```python
from build123d import *

# Parameters (mm, degrees)
F0_W     = 10
F0_H     = 15
F0_R     = 6
F0_R_2   = 3
F1_DEPTH = 20
F2_DEPTH = 75
F3_DEPTH = 10
F4_R     = 3
F5_DEPTH = 113.001
F6_R     = 5


with BuildPart() as f1:
    # F0 (on Top) → F1 (new body)
    with BuildSketch(Plane.XY):
        with Locations((-51.5, 0)):
            Rectangle(F0_W, F0_H)
        with BuildLine():
            ThreePointArc((-15.8113883008, -7.5), (-17.5, 0), (-15.8113883008, 7.5))
            Line((-15.8113883008, 7.5), (-46.5, 7.5))
            Line((-46.5, 7.5), (-46.5, -7.5))
            Line((-46.5, -7.5), (-15.8113883008, -7.5))
        make_face()
        with BuildLine():
            ThreePointArc((15.8113883008, -7.5), (17.0726286093, -3.843872054), (17.5, 0))
            ThreePointArc((17.5, 0), (17.0726286093, 3.843872054), (15.8113883008, 7.5))
            Line((15.8113883008, 7.5), (-15.8113883008, 7.5))
            ThreePointArc((-15.8113883008, 7.5), (-17.5, 0), (-15.8113883008, -7.5))
            Line((-15.8113883008, -7.5), (15.8113883008, -7.5))
        make_face()
        Circle(F0_R, mode=Mode.SUBTRACT)
        with BuildLine():
            Line((-15.8113883008, 7.5), (15.8113883008, 7.5))
            ThreePointArc((15.8113883008, 7.5), (0, 17.5), (-15.8113883008, 7.5))
        make_face()
        with BuildLine():
            ThreePointArc((-15.8113883008, -7.5), (0, -17.5), (15.8113883008, -7.5))
            Line((15.8113883008, -7.5), (-15.8113883008, -7.5))
        make_face()
        Circle(F0_R)
        Circle(F0_R_2, mode=Mode.SUBTRACT)
        with BuildLine():
            ThreePointArc((15.8113883008, 7.5), (17.0726286093, 3.843872054), (17.5, 0))
            ThreePointArc((17.5, 0), (17.0726286093, -3.843872054), (15.8113883008, -7.5))
            Line((15.8113883008, -7.5), (46.5, -7.5))
            Line((46.5, -7.5), (46.5, 7.5))
            Line((46.5, 7.5), (15.8113883008, 7.5))
        make_face()
        with Locations((51.5, 0)):
            Rectangle(F0_W, F0_H)
    extrude(amount=F1_DEPTH)

    # F0 (on Top) → F2 (join)
    with BuildSketch(Plane.XY):
        with Locations((-51.5, 0)):
            Rectangle(F0_W, F0_H)
        with Locations((51.5, 0)):
            Rectangle(F0_W, F0_H)
    extrude(amount=-F2_DEPTH)

    # F0 (on Top) → F3 (cut)
    with BuildSketch(Plane.XY):
        Circle(F0_R)
        Circle(F0_R_2, mode=Mode.SUBTRACT)
    extrude(amount=F3_DEPTH, mode=Mode.SUBTRACT)

    # F4 (on face) → F5 (cut, through all)
    with BuildSketch(Plane.YZ.offset(56.5)):
        with BuildLine():
            Line((7.5, -75), (7.5, -67.5))
            ThreePointArc((7.5, -67.5), (5.3033008589, -72.8033008589), (0, -75))
            Line((0, -75), (7.5, -75))
        make_face()
        with BuildLine():
            Line((-7.5, -75), (0, -75))
            ThreePointArc((0, -75), (-5.3033008589, -72.8033008589), (-7.5, -67.5))
            Line((-7.5, -67.5), (-7.5, -75))
        make_face()
        with Locations((0, -67.5)):
            Circle(F4_R)
    extrude(amount=-F5_DEPTH, mode=Mode.SUBTRACT)

    # F6
    f6_edges = [f1.edges().sort_by_distance(p)[0] for p in [
        (-36.155694, -7.5, 20),
        (-56.5, -7.5, -23.75),
        (56.5, -7.5, -23.75),
        (36.155694, -7.5, 20),
        (56.5, 0, 20),
        (-56.5, 0, 20),
        (-36.155694, 7.5, 20),
        (36.155694, 7.5, 20),
        (0, -17.5, 0),
        (-31.155694, -7.5, 0),
        (31.155694, -7.5, 0),
        (-31.155694, 7.5, 0),
        (31.155694, 7.5, 0),
        (0, 17.5, 0),
    ]]
    fillet(f6_edges, radius=F6_R)


solid = f1.part
```
Here's how the part is built. I have some questions about the finished solid (model axes, mm). A direction names the side the tool comes from. Round coordinates to 2 decimals unless told otherwise and drop trailing zeros. Loops run counter-clockwise (first coordinate to the right, second up) from the corner with the lowest first, then second, coordinate; pieces in that order, holes last.
1. For faces 1 (the face through (29.13, 6, 1.43)), 2 (the face through (47, 7.5, -14)), 3 (the face through (-47, -7.5, -14)), which set-ups out of +Z, -Z, +X, -X, +Y, -Y let a thin tool reach every point of the face, with its end or its side?
Answers:
face 1: -Z, +Y
face 2: +Z, -Z, +X, +Y
face 3: +Z, -Z, -X, -Y
2. Thinking about a two-plate mould opening in Y: for faces 4 (the face through (-29.13, -6, 1.43)), 5 (the face through (-3, -1, 10)), 6 (the face through (0.35, 17.497, 12.395)), which applies, released by +Y, released by -Y, zero draft, split by the parting line, or undercut?
Answers:
face 4: released by -Y
face 5: undercut
face 6: released by +Y
3. Suppose I cut it at B-B, the plane z = -59.5. Please give me the cut outline in (x, y).
Answers:
outline: (-56.5, -2.5) arc R5 ccw to (-51.5, -7.5) - (-46.5, -7.5) - (-46.5, 7.5) - (-51.5, 7.5) arc R5 ccw to (-56.5, 2.5) - close; (46.5, -7.5) - (51.5, -7.5) arc R5 ccw to (56.5, -2.5) - (56.5, 2.5) arc R5 ccw to (51.5, 7.5) - (46.5, 7.5) - close
4. Suppose I cut it at A-A, the plane x = 0. Please give me the cut outline in (y, z), and give its area (3 significant figures).
Answers:
outline: (-17.5, 5) arc R5 ccw to (-12.5, 0) - (-6, 0) - (-6, 10) - (-3, 10) - (-3, 20) - (-17.5, 20) - close; (3, 10) - (6, 10) - (6, 0) - (12.5, 0) arc R5 ccw to (17.5, 5) - (17.5, 20) - (3, 20) - close
area: 509 mm2
5. Will these pins go through, and if not, where does the flat tip stop? pin 1 (9.5 mm diameter, centred on y = 0, z = -67.5, fed in from +X); pin 2 (5 mm diameter, centred on y = 0, z = -67.5, fed in from +X); pin 3 (6 mm diameter, centred on x = 43, y = -1.5, fed in from -Z); pin 4 (6 mm diameter, centred on y = -9.5, z = 0, fed in from +X).
Answers:
pin 1: stops at x = 56.5
pin 2: passes through
pin 3: stops at z = 0
pin 4: stops at x = 54.5
6. Suppose I cut it at D-D, the plane x = 26. Please give me the cut outline in (y, z), and give its area (3 significant figures).
Answers:
outline: (-7.5, 5) arc R5 ccw to (-2.5, 0) - (2.5, 0) arc R5 ccw to (7.5, 5) - (7.5, 15) arc R5 ccw to (2.5, 20) - (-2.5, 20) arc R5 ccw to (-7.5, 15) - close
area: 279 mm2
7. Suppose I cut it at C-C, the plane z = 7. Please give me the cut outline in (x, y).
Answers:
outline: (-56.5, -2.5) arc R5 ccw to (-51.5, -7.5) - (-15.81, -7.5) arc R17.5 ccw to (15.81, -7.5) - (51.5, -7.5) arc R5 ccw to (56.5, -2.5) - (56.5, 2.5) arc R5 ccw to (51.5, 7.5) - (15.81, 7.5) arc R17.5 ccw to (-15.81, 7.5) - (-51.5, 7.5) arc R5 ccw to (-56.5, 2.5) - close; hole circle Ø12 at (0, 0)
8. If I drill on probe 1 along Y at (x, z) = (0, 13.5); probe 2 along Z at (x, y) = (-49, 0); probe 3 along Y at (x, z) = (-49, -67.5), over which ranges is the centre line in solid material (lowest first)?
Answers:
probe 1: y = -17.5 to -3, 3 to 17.5
probe 2: z = -75 to -70.5, -64.5 to 20
probe 3: y = -7.5 to -3, 3 to 7.5
